Input: part model. Units: mm. Frame: model coordinates. Face numbers are marked on the shaded views. A direction names the side the tool comes from. Give positions to 0.01 mm unless a question says otherwise; leave off trailing zeros. Write each loop counter-clockwise with the first axis right and the second up, starting at its lowest first coordinate (ties: lowest second). Pieces come first, ordered by that corner, then holes. Notation, with made-up numbers: M 48.25,66 L 54.25,66 A24 cw 54.25,97 Z; hole C -11,30.5 d2. An arc over 180 degrees is marked long. Use CSV: the item, a comma, the result in double quotes. Start each with the question number.
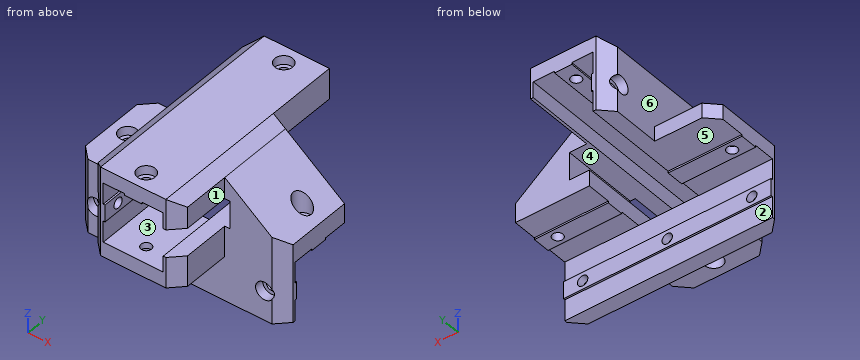
from build123d import *

# Parameters (mm, degrees)
EXTRUDE_1_DEPTH          = 22
CUT_EXTRUDE_2_DEPTH      = 82.358095651
SKETCH_3_W               = 24.9
SKETCH_3_H               = 5.8
EXTRUDE_2_DEPTH          = 0.6
CUT_EXTRUDE_3_DEPTH      = 57.272077989
EXTRUDE_3_DEPTH          = 20
CUT_EXTRUDE_4_DEPTH      = 57.272077989
CUT_EXTRUDE_4_DEPTH_BACK = 57.272077989
SKETCH_7_W               = 19.9
SKETCH_7_H               = 17
CUT_EXTRUDE_5_DEPTH      = 65.954905342
SKETCH_8_W               = 15
SKETCH_8_H               = 20
CUT_EXTRUDE_6_DEPTH      = 67.643957215
CUT_EXTRUDE_7_DEPTH      = 57.509351096
CUT_EXTRUDE_7_DEPTH_BACK = 57.509351096
SKETCH_9_R               = 1.75
SKETCH_10_R              = 1.75
CUT_EXTRUDE_8_DEPTH      = 63.543241308
SKETCH_11_W              = 0.9
SKETCH_11_H              = 24
CUT_EXTRUDE_9_DEPTH      = 10
EXTRUDE_4_DEPTH          = 70
SKETCH_13_W              = 4.1
SKETCH_13_H              = 24
CUT_EXTRUDE_10_DEPTH     = 67.682432179
SKETCH_14_R              = 1.75
CUT_EXTRUDE_11_DEPTH     = 66.197444438
SKETCH_15_W              = 5.8
SKETCH_15_H              = 0.6
EXTRUDE_5_DEPTH          = 70
SKETCH_16_R              = 1.75
CUT_EXTRUDE_12_DEPTH     = 63.05183098
EXTRUDE_START            = -26
EXTRUDE_6_DEPTH          = 26
SKETCH_18_R              = 1.75
CUT_EXTRUDE_13_DEPTH     = 58.511275079
SKETCH_20_R              = 3
CUT_EXTRUDE_17_DEPTH     = 3
SKETCH_21_R              = 3
CUT_EXTRUDE_18_DEPTH     = 20
SKETCH_22_R              = 3
CUT_EXTRUDE_19_DEPTH     = 3
SKETCH_23_R              = 3
CUT_EXTRUDE_20_DEPTH     = 3
CUT_EXTRUDE_START        = -3
SKETCH_24_R              = 3
CUT_EXTRUDE_21_DEPTH     = 3
SKETCH_25_R              = 3
CUT_EXTRUDE_22_DEPTH     = 3
SKETCH_26_W              = 6.7
SKETCH_26_H              = 9.4
CUT_EXTRUDE_23_DEPTH     = 83.281101889


with BuildPart() as part:
    # 草图1 → 凸台-拉伸1 (new body)
    with BuildSketch(Plane.XY):
        Polygon((-34.855445258, 14.044802973), (-10.855445258, 38.044802973), (11.144554742, 38.044802973), (35.144554742, 14.044802973), (35.144554742, -7.955197027), (11.144554742, -31.955197027), (-10.855445258, -31.955197027), (-34.855445258, -7.955197027), align=None)
    extrude(amount=EXTRUDE_1_DEPTH)

    # 草图2 → 切除-拉伸2 (cut, through all)
    with BuildSketch(Plane(origin=(0, 38.044802973, 0), x_dir=(1, 0, 0), z_dir=(0, 1, 0))):
        Polygon((10.244554742, 0), (-9.955445258, 0), (-9.955445258, -7.2), (-9.355445258, -7.2), (-9.355445258, -13), (-9.955445258, -13), (-9.955445258, -20.2), (-2.755445258, -20.2), (-2.755445258, -19.6), (3.044554742, -19.6), (3.044554742, -20.2), (10.244554742, -20.2), (10.244554742, -14.8), (16.944554742, -14.8), (16.944554742, -5.4), (10.244554742, -5.4), align=None)
    extrude(amount=-CUT_EXTRUDE_2_DEPTH, mode=Mode.SUBTRACT)

    # 草图3 → 凸台-拉伸2 (add)
    with BuildSketch(Plane(origin=(0, 0, 0), x_dir=(-1, 0, 0), z_dir=(0, 0, -1))):
        with Locations((22.405445258, 3.044802973)):
            Rectangle(SKETCH_3_W, SKETCH_3_H)
        with Locations((-22.694554742, 3.044802973)):
            Rectangle(SKETCH_3_W, SKETCH_3_H)
    extrude(amount=EXTRUDE_2_DEPTH)

    # 草图4 → 切除-拉伸3 (cut, through all)
    with BuildSketch(Plane(origin=(0, 0, 0), x_dir=(-1, 0, 0), z_dir=(0, 0, -1))):
        Polygon((-35.144554742, 14.044802973), (-11.144554742, 38.044802973), (-11.144554742, 14.044802973), align=None)
    extrude(amount=-CUT_EXTRUDE_3_DEPTH, mode=Mode.SUBTRACT)

    # 草图5 → 凸台-拉伸3 (add)
    with BuildSketch(Plane(origin=(0, 0, 0), x_dir=(-1, 0, 0), z_dir=(0, 0, -1))):
        Polygon((-11.144554742, -31.955197027), (10.855445258, -31.955197027), (34.855445258, -7.955197027), (34.855445258, -7.055197027), (-35.144554742, -7.055197027), (-35.144554742, -7.955197027), align=None)
    extrude(amount=EXTRUDE_3_DEPTH)

    # 草图6 → 切除-拉伸4 (cut, two sides: drawn at the far end of the back side and taken through both)
    with BuildSketch(Plane(origin=(0, 0, 0), x_dir=(-1, 0, 0), z_dir=(0, 0, -1)).offset(-CUT_EXTRUDE_4_DEPTH_BACK)):
        Polygon((14.955445258, 33.944802973), (30.855445258, 18.044802973), (14.955445258, 18.044802973), align=None)
        Polygon((14.955445258, -11.955197027), (30.855445258, -11.955197027), (14.955445258, -27.855197027), align=None)
        Polygon((-15.244554742, -11.955197027), (-31.144554742, -11.955197027), (-15.244554742, -27.855197027), align=None)
    extrude(amount=CUT_EXTRUDE_4_DEPTH + CUT_EXTRUDE_4_DEPTH_BACK, mode=Mode.SUBTRACT)

    # 草图7 → 切除-拉伸5 (cut, through all)
    with BuildSketch(Plane(origin=(0, 18.044802973, 0), x_dir=(1, 0, 0), z_dir=(0, 1, 0))):
        with Locations((-24.905445258, -13.5)):
            Rectangle(SKETCH_7_W, SKETCH_7_H)
        with Locations((25.194554742, -13.5)):
            Rectangle(SKETCH_7_W, SKETCH_7_H)
    extrude(amount=-CUT_EXTRUDE_5_DEPTH, mode=Mode.SUBTRACT)

    # 草图8 → 切除-拉伸6 (cut, through all)
    with BuildSketch(Plane.ZY.offset(14.955445258)):
        with Locations((-12.5, -21.955197027)):
            Rectangle(SKETCH_8_W, SKETCH_8_H)
    extrude(amount=-CUT_EXTRUDE_6_DEPTH, mode=Mode.SUBTRACT)

    # 草图9 → 切除-拉伸7 (cut, two sides: drawn at the far end of the back side and taken through both)
    with BuildSketch(Plane(origin=(0, 0, -0.6), x_dir=(-1, 0, 0), z_dir=(0, 0, -1)).offset(-CUT_EXTRUDE_7_DEPTH_BACK)):
        with Locations((-29.544554742, 3.044802973)):
            Circle(SKETCH_9_R)
        with Locations((29.255445258, 3.044802973)):
            Circle(SKETCH_9_R)
        with Locations((-0.144554742, 32.444802973)):
            Circle(SKETCH_9_R)
        with Locations((-0.144554742, -26.355197027)):
            Circle(SKETCH_9_R)
    extrude(amount=CUT_EXTRUDE_7_DEPTH + CUT_EXTRUDE_7_DEPTH_BACK, mode=Mode.SUBTRACT)

    # 草图10 → 切除-拉伸8 (cut, through all)
    with BuildSketch(Plane(origin=(-9.355445258, 0, 0), x_dir=(0, 0, -1), z_dir=(1, 0, 0))):
        with Locations((-10.1, 32.444802973)):
            Circle(SKETCH_10_R)
        with Locations((-10.1, -26.355197027)):
            Circle(SKETCH_10_R)
        with Locations((-10.1, 3.044802973)):
            Circle(SKETCH_10_R)
    extrude(amount=-CUT_EXTRUDE_8_DEPTH, mode=Mode.SUBTRACT)

    # 草图11 → 切除-拉伸9 (cut)
    with BuildSketch(Plane(origin=(0, 0, 0), x_dir=(-1, 0, 0), z_dir=(0, 0, -1))):
        with Locations((-10.694554742, 26.044802973)):
            Rectangle(SKETCH_11_W, SKETCH_11_H)
    extrude(amount=-CUT_EXTRUDE_9_DEPTH, mode=Mode.SUBTRACT)

    # 草图12 → 凸台-拉伸4 (add)
    with BuildSketch(Plane(origin=(0, 38.044802973, 0), x_dir=(1, 0, 0), z_dir=(0, 1, 0))):
        Polygon((-14.955445258, -22), (-10.855445258, -25.2), (11.144554742, -25.2), (15.244554742, -22), align=None)
    extrude(amount=-EXTRUDE_4_DEPTH)

    # 草图13 → 切除-拉伸10 (cut, through all)
    with BuildSketch(Plane(origin=(0, 0, 22), x_dir=(-1, 0, 0), z_dir=(0, 0, -1))):
        Polygon((10.855445258, 38.044802973), (14.955445258, 38.044802973), (14.955445258, 33.944802973), align=None)
        with Locations((-13.194554742, 26.044802973)):
            Rectangle(SKETCH_13_W, SKETCH_13_H)
        Polygon((14.955445258, -27.855197027), (14.955445258, -31.955197027), (10.855445258, -31.955197027), align=None)
        Polygon((-15.244554742, -31.955197027), (-11.144554742, -31.955197027), (-15.244554742, -27.855197027), align=None)
    extrude(amount=-CUT_EXTRUDE_10_DEPTH, mode=Mode.SUBTRACT)

    # 草图14 → 切除-拉伸11 (cut, through all)
    with BuildSketch(Plane(origin=(0, 0, 19.6), x_dir=(-1, 0, 0), z_dir=(0, 0, -1))):
        with Locations((-0.144554742, 32.444802973)):
            Circle(SKETCH_14_R)
        with Locations((-0.144554742, -26.355197027)):
            Circle(SKETCH_14_R)
    extrude(amount=-CUT_EXTRUDE_11_DEPTH, mode=Mode.SUBTRACT)

    # 草图15 → 凸台-拉伸5 (add)
    with BuildSketch(Plane.ZY.offset(34.855445258)):
        with Locations((-10, -6.755197027)):
            Rectangle(SKETCH_15_W, SKETCH_15_H)
    extrude(amount=-EXTRUDE_5_DEPTH)

    # 草图16 → 切除-拉伸12 (cut, through all)
    with BuildSketch(Plane(origin=(0, -6.455197027, 0), x_dir=(1, 0, 0), z_dir=(0, 1, 0))):
        with Locations(Location((-28.355445258, 10, 0), (0, 0, 180))):
            Circle(SKETCH_16_R)
        with Locations(Location((28.644554742, 10, 0), (0, 0, 180))):
            Circle(SKETCH_16_R)
        with Locations(Location((0.144554742, 10, 0), (0, 0, 180))):
            Circle(SKETCH_16_R)
    extrude(amount=-CUT_EXTRUDE_12_DEPTH, mode=Mode.SUBTRACT)

    # 草图17 → 凸台-拉伸6 (add)
    with BuildSketch(Plane(origin=(0, 14.044802973, 0), x_dir=(1, 0, 0), z_dir=(0, 1, 0)).offset(EXTRUDE_START)):
        Polygon((15.244554742, -5), (15.244554742, -22), (35.144554742, -6.468292683), (35.144554742, -5), align=None)
    extrude(amount=EXTRUDE_6_DEPTH)

    # 草图18 → 切除-拉伸13 (cut, through all)
    with BuildSketch(Plane(origin=(0, 0, 5), x_dir=(-1, 0, 0), z_dir=(0, 0, -1))):
        with Locations((-29.544554742, 3.044802973)):
            Circle(SKETCH_18_R)
        Polygon((-35.144554742, -11.955197027), (-35.144554742, -7.955197027), (-31.144554742, -11.955197027), align=None)
    extrude(amount=-CUT_EXTRUDE_13_DEPTH, mode=Mode.SUBTRACT)

    # 草图20 → 切除-拉伸17 (cut)
    with BuildSketch(Plane.XY.offset(25.2)):
        with Locations((0.144554742, 32.444802973)):
            Circle(SKETCH_20_R)
        with Locations((0.144554742, -26.355197027)):
            Circle(SKETCH_20_R)
    extrude(amount=-CUT_EXTRUDE_17_DEPTH, mode=Mode.SUBTRACT)

    # 草图21 → 切除-拉伸18 (cut)
    with BuildSketch(Plane.XY.offset(25.2)):
        with Locations((29.544554742, 3.044802973)):
            Circle(SKETCH_21_R)
    extrude(amount=-CUT_EXTRUDE_18_DEPTH, mode=Mode.SUBTRACT)

    # 草图22 → 切除-拉伸19 (cut)
    with BuildSketch(Plane.ZY.offset(14.955445258)):
        with Locations(Location((10.1, 32.444802973, 0), (0, 0, 270))):
            Circle(SKETCH_22_R)
        with Locations(Location((10.1, 3.044802973, 0), (0, 0, 270))):
            Circle(SKETCH_22_R)
        with Locations(Location((10.1, -26.355197027, 0), (0, 0, 270))):
            Circle(SKETCH_22_R)
    extrude(amount=-CUT_EXTRUDE_19_DEPTH, mode=Mode.SUBTRACT)

    # 草图23 → 切除-拉伸20 (cut)
    with BuildSketch(Plane.XZ.offset(11.955197027)):
        with Locations(Location((-28.355445258, -10, 0), (0, 0, 270))):
            Circle(SKETCH_23_R)
        with Locations(Location((0.144554742, -10, 0), (0, 0, 270))):
            Circle(SKETCH_23_R)
        with Locations(Location((28.644554742, -10, 0), (0, 0, 270))):
            Circle(SKETCH_23_R)
    extrude(amount=-CUT_EXTRUDE_20_DEPTH, mode=Mode.SUBTRACT)

    # 草图24 → 切除-拉伸21 (cut)
    with BuildSketch(Plane(origin=(0, 0, -5), x_dir=(-1, 0, 0), z_dir=(0, 0, -1)).offset(CUT_EXTRUDE_START)):
        with Locations(Location((-0.144554742, -26.355197027, 0), (0, 0, 180))):
            Circle(SKETCH_24_R)
    extrude(amount=CUT_EXTRUDE_21_DEPTH, mode=Mode.SUBTRACT)

    # 草图25 → 切除-拉伸22 (cut)
    with BuildSketch(Plane.XY.offset(5)):
        with Locations((-29.255445258, 3.044802973)):
            Circle(SKETCH_25_R)
    extrude(amount=-CUT_EXTRUDE_22_DEPTH, mode=Mode.SUBTRACT)

    # 草图26 → 切除-拉伸23 (cut, through all)
    with BuildSketch(Plane(origin=(0, 38.044802973, 0), x_dir=(1, 0, 0), z_dir=(0, 1, 0))):
        with Locations((13.594554742, -10.1)):
            Rectangle(SKETCH_26_W, SKETCH_26_H)
    extrude(amount=-CUT_EXTRUDE_23_DEPTH, mode=Mode.SUBTRACT)


solid = part.part
Q1. Section B-B, the plane y = -17. Return the cut outline in (x, z), and give its area (3 significant figures).
Q2. Set-up query: the marked faces 1, 2 and 3. Return all of +Z, -Z, +X, -X, +Y, -Y with unobstructed straight access to the full face (end or side cutting, diameter ignored); none if empty.
Q3. Pull-direction query (Z, two-part tool) for the marked faces 4, 5 and 6; classes: released by +Z, released by -Z, zero draft, split by the parting line, or undercut.
Q4. Section D-D, the plane y = 7. Return the cut outline in (x, z), and give its area (3 significant figures).
Q5. First-contact query: pin 1 Ø1 at (x, z) = (-26.5, -1.5) entering from -Y; pin 2 Ø8 at (y, z) = (22.5, -3.5) entering from -X; pin 3 Ø0.7 at (x, z) = (17.5, -0.5) entering from +Y. Flat tips, straight axial feed; report the tip coordinate or a pass-through.
Q6. Section A-A, the plane x = 7. Return the cut outline in (y, z).
Q7. Material intervals for L1, parallel to Y at x = -10.85, z = 10.1; L2, parallel to X at y = 32, z = 19.5; L3, parallel to X at y = -6.5, z = 1, sorted ascending. Write a range as [from, to].
Q8. Section C-C, the plane z = -10. Return the cut outline in (x, y), and give its area (3 significant figures).
Check result:
1,outline,"M -14.96,-5 L 15.24,-5 L 15.24,5.4 L 10.24,5.4 L 10.24,0 L -9.96,0 L -9.96,7.2 L -9.36,7.2 L -9.36,13 L -9.96,13 L -9.96,20.2 L -2.76,20.2 L -2.76,19.6 L 3.04,19.6 L 3.04,20.2 L 10.24,20.2 L 10.24,14.8 L 15.24,14.8 L 15.24,22 L 11.14,25.2 L -10.86,25.2 L -14.96,22 Z"
1,area,"451 mm²"
2,face 1,"+Z, -Z, +X, -Y"
2,face 2,"-Z, +X, -X, +Y"
2,face 3,"+Y, -Y"
3,face 4,"undercut"
3,face 5,"released by -Z"
3,face 6,"zero draft"
4,outline,"M -34.86,0 L -9.96,0 L -9.96,7.2 L -9.36,7.2 L -9.36,13 L -9.96,13 L -9.96,20.2 L -2.76,20.2 L -2.76,19.6 L 3.04,19.6 L 3.04,20.2 L 10.24,20.2 L 10.24,14.8 L 16.94,14.8 L 16.94,5.4 L 10.24,5.4 L 10.24,0 L 35.14,0 L 35.14,6.47 L 11.14,25.2 L -10.86,25.2 L -14.96,22 L -14.96,5 L -34.86,5 Z"
4,area,"667 mm²"
5,pin 1,"stops at y = -11.96"
5,pin 2,"stops at x = -14.96"
5,pin 3,"stops at y = 5.94"
6,outline,"M -31.96,-5 L -11.96,-5 L -11.96,-20 L -7.06,-20 L -7.06,-12.9 L -6.46,-12.9 L -6.46,-7.1 L -7.06,-7.1 L -7.06,0 L -31.96,0 Z; M -31.96,20.2 L 38.04,20.2 L 38.04,25.2 L -31.96,25.2 Z"
7,L1,"y = [-31.96, -28.11], [-24.61, 1.29], [4.79, 30.69], [34.19, 38.04]"
7,L2,"x = [-14.96, -9.96], [10.24, 11.14]"
7,L3,"x = [-34.86, -9.96], [10.24, 35.14]"
8,outline,"M -34.86,-7.96 L -31.36,-11.46 L -31.36,-8.96 L -30.11,-8.96 L -30.11,-6.46 L -34.86,-6.46 Z; M -26.61,-8.96 L -25.36,-8.96 L -25.36,-11.96 L -2.86,-11.96 L -2.86,-8.96 L -1.61,-8.96 L -1.61,-6.46 L -26.61,-6.46 Z; M 1.89,-8.96 L 3.14,-8.96 L 3.14,-11.96 L 25.64,-11.96 L 25.64,-8.96 L 26.89,-8.96 L 26.89,-6.46 L 1.89,-6.46 Z; M 30.39,-8.96 L 31.64,-8.96 L 31.64,-11.46 L 35.14,-7.96 L 35.14,-6.46 L 30.39,-6.46 Z"
8,area,"289 mm²"
